```python
from build123d import *

# Parameters (mm, degrees)
IZIM2_W                          = 40
IZIM2_H                          = 32
Y_KSEKLIK_EKSTR_ZYON1_DEPTH      = 9.17
IZIM3_W                          = 40
IZIM3_H                          = 1.915150366
Y_KSEKLIK_EKSTR_ZYON2_DEPTH      = 12.39
IZIM4_W                          = 10
IZIM4_H                          = 12.39
KES_EKSTR_ZYON1_DEPTH            = 12.39
Y_KSEKLIK_EKSTR_ZYON3_DEPTH      = 4
Y_KSEKLIK_EKSTR_ZYON3_DEPTH_BACK = 1.91515
IZIM5_W                          = 74.37
IZIM5_H                          = 3
IZIM6_W                          = 4.45
IZIM6_H                          = 3
Y_KSEKLIK_EKSTR_ZYON4_DEPTH      = 4.71
IZIM7_W                          = 5.92
IZIM7_H                          = 1.9
Y_KSEKLIK_EKSTR_ZYON5_DEPTH      = 74.37
RADYUS1_R                        = 3
RADYUS2_R                        = 2
RADYUS3_R                        = 1
RADYUS4_R                        = 0.5
IZIM8_R                          = 1.25
KES_EKSTR_ZYON2_DEPTH            = 10
IZIM9_R                          = 1.5
KES_EKSTR_ZYON3_DEPTH            = 10


with BuildPart() as part:
    # Çizim2 → Yükseklik-Ekstrüzyon1 (new body)
    with BuildSketch(Plane(origin=(0, 0, 0), x_dir=(1, 0, 0), z_dir=(0, 1, 0))):
        Rectangle(IZIM2_W, IZIM2_H)
    extrude(amount=Y_KSEKLIK_EKSTR_ZYON1_DEPTH)

    # Çizim3 → Yükseklik-Ekstrüzyon2 (add)
    with BuildSketch(Plane(origin=(0, 0, 0), x_dir=(-1, 0, 0), z_dir=(0, -1, 0))):
        with Locations((0, -15.042424817)):
            Rectangle(IZIM3_W, IZIM3_H)
    extrude(amount=Y_KSEKLIK_EKSTR_ZYON2_DEPTH)

    # Çizim4 → Kes-Ekstrüzyon1 (cut)
    with BuildSketch(Plane.XY.offset(16)):
        with Locations((-15, -6.195)):
            Rectangle(IZIM4_W, IZIM4_H)
        with Locations((15, -6.195)):
            Rectangle(IZIM4_W, IZIM4_H)
    extrude(amount=-KES_EKSTR_ZYON1_DEPTH, mode=Mode.SUBTRACT)

    # Çizim5 → Yükseklik-Ekstrüzyon3 (add, two sides: drawn at the far end of the back side and taken through both)
    with BuildSketch(Plane.XY.offset(16).offset(-Y_KSEKLIK_EKSTR_ZYON3_DEPTH_BACK)):
        with Locations((0, -12.39)):
            Rectangle(IZIM5_W, IZIM5_H)
    extrude(amount=Y_KSEKLIK_EKSTR_ZYON3_DEPTH + Y_KSEKLIK_EKSTR_ZYON3_DEPTH_BACK)

    # Çizim6 → Yükseklik-Ekstrüzyon4 (add)
    with BuildSketch(Plane.XY.offset(20)):
        with Locations((-34.96, -12.39)):
            Rectangle(IZIM6_W, IZIM6_H)
        with Locations((34.96, -12.39)):
            Rectangle(IZIM6_W, IZIM6_H)
    extrude(amount=Y_KSEKLIK_EKSTR_ZYON4_DEPTH)

    # Çizim7 → Yükseklik-Ekstrüzyon5 (add)
    with BuildSketch(Plane(origin=(37.185, 0, 0), x_dir=(0, 0, -1), z_dir=(1, 0, 0))):
        with Locations((-17.044849634, -14.84)):
            Rectangle(IZIM7_W, IZIM7_H)
    extrude(amount=-Y_KSEKLIK_EKSTR_ZYON5_DEPTH)

    # Radyus1
    radyus1_edges = [part.edges().sort_by_distance(p)[0] for p in [
        (-10, -10.89, 15.042425),
        (10, -10.89, 15.042425),
    ]]
    fillet(radyus1_edges, radius=RADYUS1_R)

    # Radyus2
    radyus2_edges = [part.edges().sort_by_distance(p)[0] for p in [
        (-10, 0, 15.042424817),
        (10, 0, 15.042424817),
    ]]
    fillet(radyus2_edges, radius=RADYUS2_R)

    # Radyus3
    radyus3_edges = [part.edges().sort_by_distance(p)[0] for p in [
        (-20, 4.585, -16),
        (20, 4.585, -16),
        (20, 4.585, 16),
        (-20, 4.585, 16),
    ]]
    fillet(radyus3_edges, radius=RADYUS3_R)

    # Radyus4
    # the kernel refuses this fillet: 0.5 mm, written as the material it adds along each edge
    with BuildSketch(Plane(origin=(-32.735, -10.89, 20), x_dir=(1, 0, 0), z_dir=(0, -1, 0)), Plane(origin=(32.735, -10.89, 20), x_dir=(0, 0, 1), z_dir=(0, -1, 0))) as radyus4_piece_1:
        with BuildLine():
            CenterArc((RADYUS4_R, RADYUS4_R), RADYUS4_R, 180, 90)
            Line((0, RADYUS4_R), (0, 0))
            Line((0, 0), (RADYUS4_R, 0))
        make_face()
    extrude(amount=3)

    # Çizim8 → Kes-Ekstrüzyon2 (cut)
    with BuildSketch(Plane(origin=(0, -10.89, 0), x_dir=(1, 0, 0), z_dir=(0, 1, 0))):
        with Locations(Location((-34.765, -22.5, 0), (0, 0, 180))):
            Circle(IZIM8_R)
        with Locations(Location((34.735, -22.5, 0), (0, 0, 180))):
            Circle(IZIM8_R)
    extrude(amount=-KES_EKSTR_ZYON2_DEPTH, mode=Mode.SUBTRACT)

    # Çizim9 → Kes-Ekstrüzyon3 (cut)
    with BuildSketch(Plane(origin=(0, 9.17, 0), x_dir=(1, 0, 0), z_dir=(0, 1, 0))):
        with Locations(Location((-16, -9.08, 0), (0, 0, 270))):
            Circle(IZIM9_R)
        with Locations(Location((-16, 11, 0), (0, 0, 270))):
            Circle(IZIM9_R)
        with Locations(Location((16, 11, 0), (0, 0, 270))):
            Circle(IZIM9_R)
        with Locations(Location((16, -9.08, 0), (0, 0, 270))):
            Circle(IZIM9_R)
    extrude(amount=-KES_EKSTR_ZYON3_DEPTH, mode=Mode.SUBTRACT)


solid = part.part
```
Input: part model. Units: mm. Frame: model coordinates. A direction names the side the tool comes from. Coordinates: 2 decimals unless noted, no trailing zeros. Write each loop counter-clockwise with the first axis right and the second up, starting at its lowest first coordinate (ties: lowest second). Pieces come first, ordered by that corner, then holes.
1) Pin query (flat end, axial travel): pin 1 Ø3 at (y, z) = (-3.5, 17) entering from -X; pin 2 Ø3 at (y, z) = (2.5, -3.5) entering from -X; pin 3 Ø3 at (y, z) = (3.5, -11) entering from +X; pin 4 Ø12 at (y, z) = (-9.5, -7) entering from -X. Return the tip coordinate at first contact, or that it passes through.
2) Mould query, pull axis Y, two halves, no side actions, for faces 4 (the cylindrical face through (10.6, -0.57, 15.03)), 5 (the flat face through (35, -12, 24.71)), 6 (the flat face through (1, -15.79, 17)), 7 (the flat face through (10, -5, 15)). Classes: pulls with the +Y half, pulls with the -Y half, needs draft (parallel to the pull), parting line crosses it, or undercut.
3) Section D-D on y = 4. Output: boundary loops of the cut face in (x, z), and give its area (3 significant figures).
4) Material intervals for line 1 along X through (y, z) = (2.5, 9.08); line 2 along Z through (x, y) = (0, -2.75); line 3 along Z through (x, y) = (-6, -14.25), sorted ascending.
5) Section C-C on z = -11. Output: boundary loops of the cut face in (x, y), and give its area (3 significant figures).
6) Section B-B on z = 22.5. Output: boundary loops of the cut face in (x, y) (3 decimals).
7) Set-up query: faces 1 (the flat face through (-32.735, -12, 23)), 2 (the flat face through (0, 2, 16)), 3 (the flat face through (35, -13.89, 21)). Return all of +Z, -Z, +X, -X, +Y, -Y with unobstructed straight access to the full face (end or side cutting, diameter ignored); none if empty.
8) Section A-A on x = -16. State how many separate pieces and enclosed holes the cut face has, and give its area (3 significant figures).
Check result:
1. pin 1: stops at x = -10
1. pin 2: stops at x = -20
1. pin 3: stops at x = 20
1. pin 4: passes through
2. face 4: undercut
2. face 5: needs draft
2. face 6: pulls with the -Y half
2. face 7: undercut
3. outline: (-20, -15) arc R1 ccw to (-19, -16) - (19, -16) arc R1 ccw to (20, -15) - (20, 15) arc R1 ccw to (19, 16) - (-19, 16) arc R1 ccw to (-20, 15) - close; hole circle Ø3 at (-16, -11); hole circle Ø3 at (-16, 9.08); hole circle Ø3 at (16, -11); hole circle Ø3 at (16, 9.08)
3. area: 1,250 mm2
4. line 1: x = -20 to -17.5, -14.5 to 14.5, 17.5 to 20
4. line 2: z = 14.08 to 16
4. line 3: z = 14.08 to 20
5. outline: (-20, 0) - (-17.5, 0) - (-17.5, 9.17) - (-20, 9.17) - close; (-14.5, 0) - (14.5, 0) - (14.5, 9.17) - (-14.5, 9.17) - close; (17.5, 0) - (20, 0) - (20, 9.17) - (17.5, 9.17) - close
5. area: 312 mm2
6. outline: (-37.185, -13.89) - (-36.015, -13.89) - (-36.015, -10.89) - (-37.185, -10.89) - close; (-33.515, -13.89) - (-32.735, -13.89) - (-32.735, -10.89) - (-33.515, -10.89) - close; (32.735, -13.89) - (33.485, -13.89) - (33.485, -10.89) - (32.735, -10.89) - close; (35.985, -13.89) - (37.185, -13.89) - (37.185, -10.89) - (35.985, -10.89) - close
7. face 1: +Z, +Y, -Y
7. face 2: +Z, +X, -X, +Y
7. face 3: +Z, +X, -X, -Y
8. separate pieces: 4
8. enclosed holes: 0
8. area: 267 mm2
